Source: CAD feature listing. Evaluate the final solid. Frame: model axes, mm. Face numbers are marked on the shaded views. A direction names the side the tool comes from. Round coordinates to 2 decimals unless told otherwise and drop trailing zeros. Write each loop counter-clockwise with the first axis right and the second up, starting at its lowest first coordinate (ties: lowest second). Pieces come first, ordered by that corner, then holes.
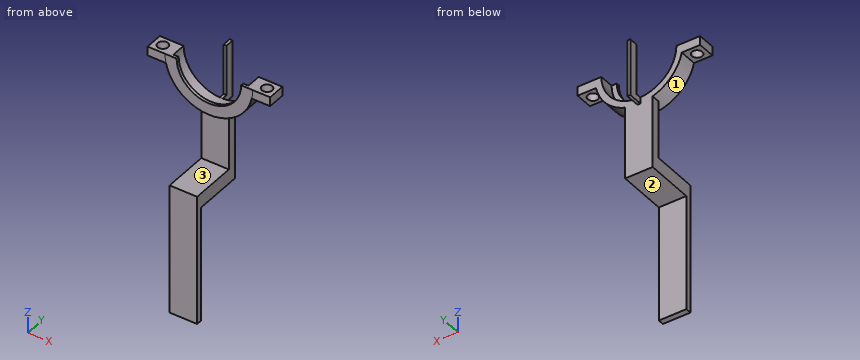
```python
from build123d import *

# Parameters (mm, degrees)
BOSS_EXTRUDE1_DEPTH = 5
BOSS_EXTRUDE2_DEPTH = 3
BOSS_EXTRUDE3_DEPTH = 3
SKETCH10_W          = 9.5
SKETCH10_H          = 5
BOSS_EXTRUDE4_DEPTH = 15.78
SKETCH11_W          = 9.5
SKETCH11_H          = 2
BOSS_EXTRUDE5_DEPTH = 40
BOSS_EXTRUDE6_DEPTH = 6.09393
SKETCH14_R          = 1.8
CUT_EXTRUDE1_DEPTH  = 6.3
SKETCH15_W          = 51.153217575
SKETCH15_H          = 31.902182189
CUT_EXTRUDE3_DEPTH  = 19.78


with BuildPart() as part:
    # Sketch3 → Revolve1 (revolve)
    with BuildSketch(Plane.XY):
        Polygon((-62.694264441, 10.250679103), (-62.694264441, 11.733728816), (-64.884531744, 11.733728816), (-64.884531744, 5.639799249), (-60.884531744, 5.639799249), (-60.884531744, 6.650679103), (-62.694264441, 6.650679103), align=None)
    revolve(axis=Axis((-49.744264441, 0, 0), (0, 1, 0)))

    # Sketch7 → Boss-Extrude1 (add)
    with BuildSketch(Plane(origin=(0, 11.733728816, 0), x_dir=(1, 0, 0), z_dir=(0, 1, 0))):
        with BuildLine():
            Line((-50.244264441, 15.132008921), (-50.244264441, 12.94034389))
            ThreePointArc((-50.244264441, 12.94034389), (-49.744264441, 12.95), (-49.244264441, 12.94034389))
            Line((-49.244264441, 12.94034389), (-49.244264441, 15.132008921))
            ThreePointArc((-49.244264441, 15.132008921), (-49.744264441, 15.140267302), (-50.244264441, 15.132008921))
        make_face()
    extrude(amount=BOSS_EXTRUDE1_DEPTH)

    # Sketch8 → Boss-Extrude2 (add)
    with BuildSketch(Plane(origin=(0, 16.733728816, 0), x_dir=(1, 0, 0), z_dir=(0, 1, 0))):
        with BuildLine():
            Line((-50.244264441, 15.132008921), (-50.244264441, 12.94034389))
            Line((-50.244264441, 12.94034389), (-50.244264441, -4.55965611))
            Line((-50.244264441, -4.55965611), (-49.244264441, -4.55965611))
            Line((-49.244264441, -4.55965611), (-49.244264441, 12.94034389))
            Line((-49.244264441, 12.94034389), (-49.244264441, 15.132008921))
            ThreePointArc((-49.244264441, 15.132008921), (-49.744264441, 15.140267302), (-50.244264441, 15.132008921))
        make_face()
    extrude(amount=-BOSS_EXTRUDE2_DEPTH)

    # Sketch9 → Boss-Extrude3 (add)
    with BuildSketch(Plane(origin=(0, 11.733728816, 0), x_dir=(1, 0, 0), z_dir=(0, 1, 0))):
        with BuildLine():
            Line((-54.494264441, 14.375854548), (-54.494264441, 39.375854548))
            Line((-54.494264441, 39.375854548), (-44.994264441, 39.375854548))
            Line((-44.994264441, 39.375854548), (-44.994264441, 14.375854548))
            ThreePointArc((-44.994264441, 14.375854548), (-47.092177082, 14.906177465), (-49.244264441, 15.132008921))
            ThreePointArc((-49.244264441, 15.132008921), (-49.744264441, 15.140267302), (-50.244264441, 15.132008921))
            ThreePointArc((-50.244264441, 15.132008921), (-52.3963518, 14.906177465), (-54.494264441, 14.375854548))
        make_face()
    extrude(amount=-BOSS_EXTRUDE3_DEPTH)

    # Sketch10 → Boss-Extrude4 (add)
    with BuildSketch(Plane.XZ.offset(-8.733728816)):
        with Locations((-49.744264441, -36.875854548)):
            Rectangle(SKETCH10_W, SKETCH10_H)
    extrude(amount=BOSS_EXTRUDE4_DEPTH)

    # Sketch11 → Boss-Extrude5 (add)
    with BuildSketch(Plane(origin=(0, 0, -39.375854548), x_dir=(-1, 0, 0), z_dir=(0, 0, -1))):
        with Locations((49.744264441, -6.046271184)):
            Rectangle(SKETCH11_W, SKETCH11_H)
    extrude(amount=BOSS_EXTRUDE5_DEPTH)

    # Sketch13 → Boss-Extrude6 (add)
    with BuildSketch(Plane(origin=(0, 11.733728816, 0), x_dir=(1, 0, 0), z_dir=(0, 1, 0))):
        with BuildLine():
            Line((-28.603997139, 3.15), (-34.935307895, 3.15))
            ThreePointArc((-34.935307895, 3.15), (-34.603997139, 0), (-34.935307895, -3.15))
            Line((-34.935307895, -3.15), (-28.603997139, -3.15))
            Line((-28.603997139, -3.15), (-28.603997139, 3.15))
        make_face()
        with BuildLine():
            Line((-70.884531744, 3.15), (-70.884531744, -3.15))
            Line((-70.884531744, -3.15), (-64.553220987, -3.15))
            ThreePointArc((-64.553220987, -3.15), (-64.884531744, 0), (-64.553220987, 3.15))
            Line((-64.553220987, 3.15), (-70.884531744, 3.15))
        make_face()
    extrude(amount=-BOSS_EXTRUDE6_DEPTH)

    # Sketch14 → Cut-Extrude1 (cut)
    with BuildSketch(Plane.XY.offset(3.15)):
        with Locations((-31.769652517, 8.686764033)):
            Circle(SKETCH14_R)
        with Locations((-67.718876365, 8.686764033)):
            Circle(SKETCH14_R)
    extrude(amount=-CUT_EXTRUDE1_DEPTH, mode=Mode.SUBTRACT)

    # Sketch15 → Cut-Extrude3 (cut, through all)
    with BuildSketch(Plane(origin=(0, 11.733728816, 0), x_dir=(1, 0, 0), z_dir=(0, 1, 0))):
        with Locations((-49.018725857, -15.951091095)):
            Rectangle(SKETCH15_W, SKETCH15_H)
    extrude(amount=-CUT_EXTRUDE3_DEPTH, mode=Mode.SUBTRACT)


solid = part.part
```
Q1. Line query: line 1 (Z direction, x = -32, y = 6.75); line 2 (X direction, y = 7, z = -37.5); line 3 (Y direction, x = -48.5, z = -33.5). Output: solid intervals per line, ascending.
Q2. Section query D-D, the plane x = -42.5. Output: boundary loops of the cut face in (y, z), and give its area (3 significant figures).
Q3. Section query B-B, the plane x = -53. Output: boundary loops of the cut face in (y, z).
Q4. Set-up query: the marked faces 1, 2 and 3. Return all of +Z, -Z, +X, -X, +Y, -Y with unobstructed straight access to the full face (end or side cutting, diameter ignored); none if empty.
Q5. Section query C-C, the plane y = -1.75. Output: boundary loops of the cut face in (x, z).
Q6. Pin query (flat end, axial travel): P1, Ø8, axis at y = 6, z = -23, coming from the -X side; P2, Ø5, axis at x = -32, y = 8.5, coming from the -Z side; P3, Ø4, axis at y = 13.5, z = -7, coming from the -X side; P4, Ø1, axis at x = -34.5, y = 3.5, coming from the +Z side. Return the tip coordinate at first contact, or that it passes through.
Q7. Section query A-A, the plane x = -32. Output: boundary loops of the cut face in (y, z), and give its area (3 significant figures).
Filled in:
1. line 1: z = -3.15 to 0
1. line 2: x = -54.49 to -44.99
1. line 3: y = 8.73 to 11.73
2. outline: (5.64, -13.29) - (11.73, -13.29) - (11.73, -10.73) - (6.65, -10.73) - (6.65, -8.46) - (5.64, -8.46) - close
2. area: 17.9 mm2
3. outline: (-7.05, -79.38) - (-5.05, -79.38) - (-5.05, -39.38) - (11.73, -39.38) - (11.73, -12.53) - (6.65, -12.53) - (6.65, -10.65) - (5.64, -10.65) - (5.64, -14.79) - (8.73, -14.79) - (8.73, -34.38) - (-7.05, -34.38) - close
4. face 1: -Y
4. face 2: -Z, +X, -X, +Y
4. face 3: +X, -X, -Y
5. outline: (-54.49, -39.38) - (-44.99, -39.38) - (-44.99, -34.38) - (-54.49, -34.38) - close
6. P1: stops at x = -54.49
6. P2: stops at z = -3.15
6. P3: stops at x = -63.62
6. P4: passes through
7. outline: (5.64, -3.15) - (6.9, -3.15) - (6.9, 0) - (5.64, 0) - close; (10.47, -3.15) - (11.73, -3.15) - (11.73, 0) - (10.47, 0) - close
7. area: 7.95 mm2
